Here's the drawing with two shaded views (mm, measured from the low corner). I have some questions. Coordinates: 2 decimals unless noted, no trailing zeros. Write each loop counter-clockwise with the first axis right and the second up, starting at its lowest first coordinate (ties: lowest second). Pieces come first, ordered by that corner, then holes. Notation, with made-up numbers: M 0,32.5 L 35,32.5 A20 cw 35,37.5 Z; hole C -5.75,77 d5. An arc over 180 degrees is marked long. Answer as CSV lines item,"result". Start each with the question number.
Item 1: If I drill on line 1 along X through (y, z) = (0.75, 157.5), over which ranges is the centre line in solid material (lowest first)? Write a range as [from, to].
Item 2: I'm going to push flat-ended pins straight in: P1, Ø3, axis at x = 220.5, y = 2, coming from the +Z side; P2, Ø12, axis at x = 102.5, z = 170.5, coming from the -Y side; P3, Ø3, axis at y = 3, z = 17, coming from the +X side; P4, Ø3, axis at y = 3, z = 223.5, coming from the -X side. Where does each tip first touch, or does it pass through?
Item 3: Suppose I cut it at B-B, the plane x = 171. Write out the boundary of the cut face in (y, z), and give its area (3 significant figures).
Item 4: Suppose I cut it at A-A, the plane z = 92. Write out the boundary of the cut face in (x, y), and give its area (3 significant figures).
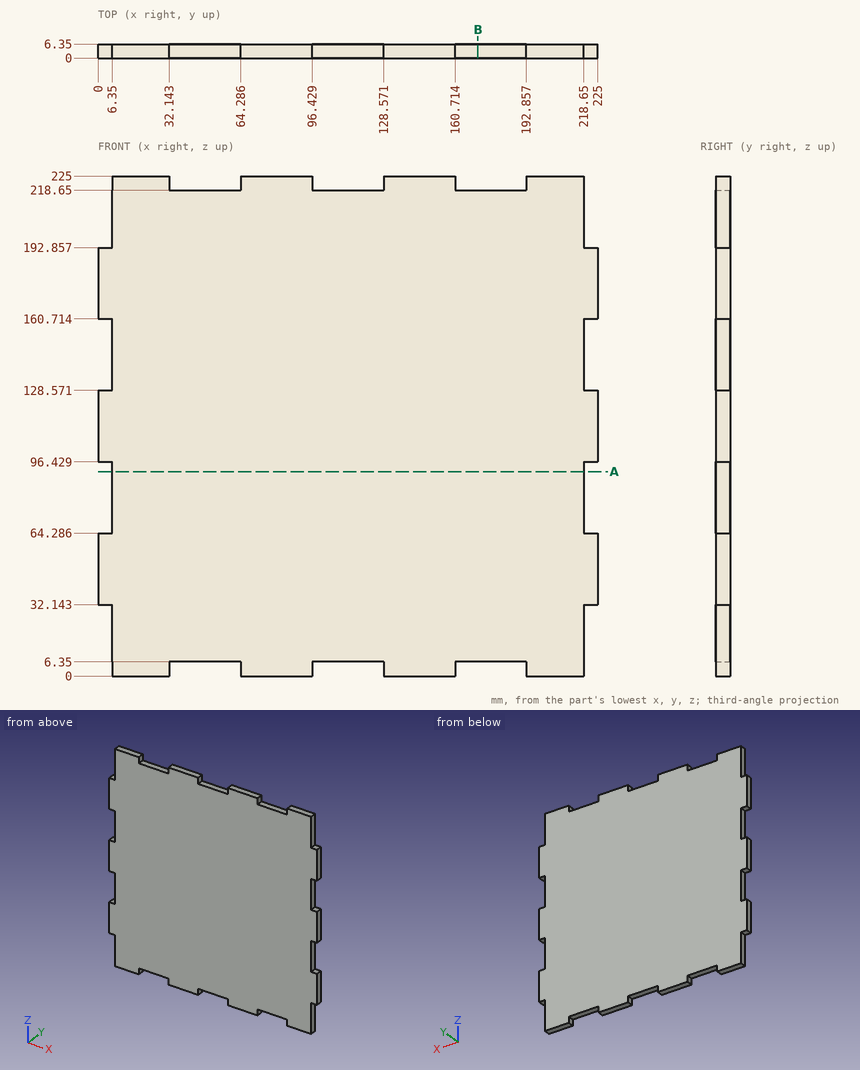
Ans:
1,line 1,"x = [6.35, 218.65]"
2,P1,"stops at z = 192.86"
2,P2,"stops at y = 0"
2,P3,"stops at x = 218.65"
2,P4,"stops at x = 6.35"
3,outline,"M 0,6.35 L 6.35,6.35 L 6.35,218.65 L 0,218.65 Z"
3,area,"1,350 mm^2"
4,outline,"M 6.35,0 L 218.65,0 L 218.65,6.35 L 6.35,6.35 Z"
4,area,"1,350 mm^2"
